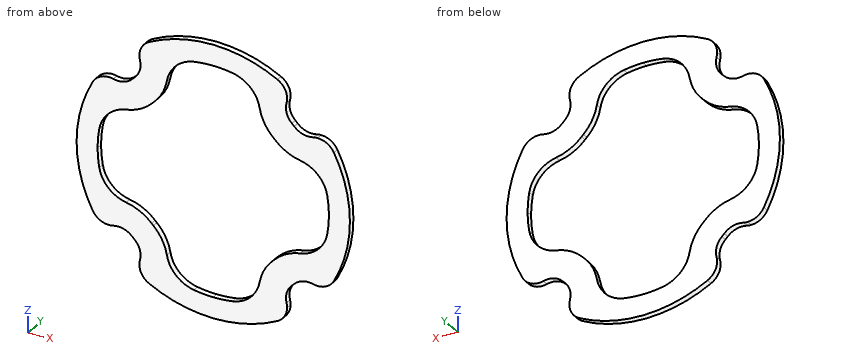
from build123d import *

# Parameters (mm, degrees)
PCB_OUTLINE_OUTER_DEPTH = 1
CUT_EXTRUDE2_DEPTH      = 1
CUT_EXTRUDE2_DEPTH_BACK = 2


with BuildPart() as part:
    # Internal Slab → PCB Outline Outer (new body)
    with BuildSketch(Plane(origin=(0, 0, 0), x_dir=(1, 0, 0), z_dir=(0, 1, 0))):
        with BuildLine():
            ThreePointArc((20.085113617, 10.68413361), (18.622288868, 12.043250737), (16.632261242, 12.207097181))
            ThreePointArc((16.632261242, 12.207097181), (14.943199752, 12.226998501), (13.492265758, 13.091935102))
            ThreePointArc((13.492265758, 13.091935102), (13.293607486, 13.293607486), (13.091935102, 13.492265758))
            ThreePointArc((13.091935102, 13.492265758), (12.226998501, 14.943199752), (12.207097181, 16.632261242))
            ThreePointArc((12.207097181, 16.632261242), (12.278791735, 17.008431368), (12.302815994, 17.390618375))
            ThreePointArc((12.302815994, 17.390618375), (11.867033623, 18.962276517), (10.68413361, 20.085113617))
            ThreePointArc((10.68413361, 20.085113617), (0, 22.75), (-10.68413361, 20.085113617))
            ThreePointArc((-10.68413361, 20.085113617), (-12.043250737, 18.622288868), (-12.207097181, 16.632261242))
            ThreePointArc((-12.207097181, 16.632261242), (-12.226998501, 14.943199752), (-13.091935102, 13.492265758))
            ThreePointArc((-13.091935102, 13.492265758), (-13.293607486, 13.293607486), (-13.492265758, 13.091935102))
            ThreePointArc((-13.492265758, 13.091935102), (-14.943199752, 12.226998501), (-16.632261242, 12.207097181))
            ThreePointArc((-16.632261242, 12.207097181), (-17.008431368, 12.278791735), (-17.390618375, 12.302815994))
            ThreePointArc((-17.390618375, 12.302815994), (-18.962276517, 11.867033623), (-20.085113617, 10.68413361))
            ThreePointArc((-20.085113617, 10.68413361), (-22.75, 0), (-20.085113617, -10.68413361))
            ThreePointArc((-20.085113617, -10.68413361), (-18.622288868, -12.043250737), (-16.632261242, -12.207097181))
            ThreePointArc((-16.632261242, -12.207097181), (-14.943199752, -12.226998501), (-13.492265758, -13.091935102))
            ThreePointArc((-13.492265758, -13.091935102), (-13.293607486, -13.293607486), (-13.091935102, -13.492265758))
            ThreePointArc((-13.091935102, -13.492265758), (-12.226998501, -14.943199752), (-12.207097181, -16.632261242))
            ThreePointArc((-12.207097181, -16.632261242), (-12.278791735, -17.008431368), (-12.302815994, -17.390618375))
            ThreePointArc((-12.302815994, -17.390618375), (-11.867033623, -18.962276517), (-10.68413361, -20.085113617))
            ThreePointArc((-10.68413361, -20.085113617), (0, -22.75), (10.68413361, -20.085113617))
            ThreePointArc((10.68413361, -20.085113617), (12.043250737, -18.622288868), (12.207097181, -16.632261242))
            ThreePointArc((12.207097181, -16.632261242), (12.226998501, -14.943199752), (13.091935102, -13.492265758))
            ThreePointArc((13.091935102, -13.492265758), (13.293607486, -13.293607486), (13.492265758, -13.091935102))
            ThreePointArc((13.492265758, -13.091935102), (14.943199752, -12.226998501), (16.632261242, -12.207097181))
            ThreePointArc((16.632261242, -12.207097181), (17.008431368, -12.278791735), (17.390618375, -12.302815994))
            ThreePointArc((17.390618375, -12.302815994), (18.962276517, -11.867033623), (20.085113617, -10.68413361))
            ThreePointArc((20.085113617, -10.68413361), (22.75, 0), (20.085113617, 10.68413361))
        make_face()
    extrude(amount=PCB_OUTLINE_OUTER_DEPTH)

    # Sketch7 → Cut-Extrude2 (cut, two sides)
    with BuildSketch(Plane(origin=(0, 1, 0), x_dir=(1, 0, 0), z_dir=(0, 1, 0))) as cut_extrude2_sk:
        with BuildLine():
            ThreePointArc((0, 19.25), (-1.616279551, 19.182026494), (-3.221144642, 18.978586017))
            ThreePointArc((-3.221144642, 18.978586017), (-6.18224043, 17.452869559), (-7.719604793, 14.497804451))
            ThreePointArc((-7.719604793, 14.497804451), (-8.503489746, 12.202965765), (-9.958227232, 10.262734061))
            ThreePointArc((-9.958227232, 10.262734061), (-10.111626971, 10.111626971), (-10.262734061, 9.958227232))
            ThreePointArc((-10.262734061, 9.958227232), (-12.202965765, 8.503489746), (-14.497804451, 7.719604793))
            ThreePointArc((-14.497804451, 7.719604793), (-17.452869559, 6.18224043), (-18.978586017, 3.221144642))
            ThreePointArc((-18.978586017, 3.221144642), (-19.182026494, 1.616279551), (-19.25, 0))
            ThreePointArc((-19.25, 0), (-19.182026494, -1.616279551), (-18.978586017, -3.221144642))
            ThreePointArc((-18.978586017, -3.221144642), (-17.452869559, -6.18224043), (-14.497804451, -7.719604793))
            ThreePointArc((-14.497804451, -7.719604793), (-12.202965765, -8.503489746), (-10.262734061, -9.958227232))
            ThreePointArc((-10.262734061, -9.958227232), (-10.111626971, -10.111626971), (-9.958227232, -10.262734061))
            ThreePointArc((-9.958227232, -10.262734061), (-8.503489746, -12.202965765), (-7.719604793, -14.497804451))
            ThreePointArc((-7.719604793, -14.497804451), (-6.18224043, -17.452869559), (-3.221144642, -18.978586017))
            ThreePointArc((-3.221144642, -18.978586017), (-1.616279551, -19.182026494), (0, -19.25))
            ThreePointArc((0, -19.25), (1.616279551, -19.182026494), (3.221144642, -18.978586017))
            ThreePointArc((3.221144642, -18.978586017), (6.18224043, -17.452869559), (7.719604793, -14.497804451))
            ThreePointArc((7.719604793, -14.497804451), (8.503489746, -12.202965765), (9.958227232, -10.262734061))
            ThreePointArc((9.958227232, -10.262734061), (10.111626971, -10.111626971), (10.262734061, -9.958227232))
            ThreePointArc((10.262734061, -9.958227232), (12.202965765, -8.503489746), (14.497804451, -7.719604793))
            ThreePointArc((14.497804451, -7.719604793), (17.452869559, -6.18224043), (18.978586017, -3.221144642))
            ThreePointArc((18.978586017, -3.221144642), (19.182026494, -1.616279551), (19.25, 0))
            ThreePointArc((19.25, 0), (19.182026494, 1.616279551), (18.978586017, 3.221144642))
            ThreePointArc((18.978586017, 3.221144642), (17.452869559, 6.18224043), (14.497804451, 7.719604793))
            ThreePointArc((14.497804451, 7.719604793), (12.202965765, 8.503489746), (10.262734061, 9.958227232))
            ThreePointArc((10.262734061, 9.958227232), (10.111626971, 10.111626971), (9.958227232, 10.262734061))
            ThreePointArc((9.958227232, 10.262734061), (8.503489746, 12.202965765), (7.719604793, 14.497804451))
            ThreePointArc((7.719604793, 14.497804451), (6.18224043, 17.452869559), (3.221144642, 18.978586017))
            ThreePointArc((3.221144642, 18.978586017), (1.616279551, 19.182026494), (0, 19.25))
        make_face()
    extrude(amount=CUT_EXTRUDE2_DEPTH, mode=Mode.SUBTRACT)
    extrude(cut_extrude2_sk.sketch, amount=-CUT_EXTRUDE2_DEPTH_BACK, mode=Mode.SUBTRACT)


solid = part.part
The listing builds one solid part. Answer for the finished solid, in the listing's coordinates (mm). Give positions to 0.01 mm unless a question says otherwise; leave off trailing zeros. Order: outer loops, then holes, each group sorted by start corner. A loop starts at its lowest first (then second) coordinate and runs counter-clockwise, first axis right, second up. Notation, with made-up numbers: (85.25, 86) - (141.25, 86) arc R31 ccw to (141.25, 119) - close; hole circle Ø3 at (-18.5, 44). An arc over 180 degrees is marked (long way). Use one line per item in the form item = value.
1) Consider probe 1 along X at (y, z) = (0.55, -6.5); probe 2 along X at (y, z) = (0.1, 1.5); probe 3 along Z at (x, y) = (-5, 0.55). Determine where each line is inside the solid, lowest interval first. Write a range as [from, to].
Verdict:
probe_1 = [-21.8, -17.11], [17.11, 21.8]
probe_2 = [-22.7, -19.19], [19.19, 22.7]
probe_3 = [-22.19, -18.35], [18.35, 22.19]
2) Find section B-B on x = -1.5. Determine the outline of the cut face in (y, z).
Verdict:
outline = (0, -22.7) - (1, -22.7) - (1, -19.19) - (0, -19.19) - close; (0, 19.19) - (1, 19.19) - (1, 22.7) - (0, 22.7) - close
3) This flat-tipped pin is pushed along its axis until it touches: pin 1 (4 mm diameter, centred on x = 4.5, z = 16, fed in from -Y). Where does it stop, or does it pass through?
Verdict:
pin_1 = through
4) Find section A-A on z = -2.5. Determine the outline of the cut face in (x, y), and give its area (3 significant figures).
Verdict:
outline = (-22.61, 0) - (-19.09, 0) - (-19.09, 1) - (-22.61, 1) - close; (19.09, 0) - (22.61, 0) - (22.61, 1) - (19.09, 1) - close
area = 7.05 mm^2
